Build history of the part. All positions in model axes, mm. Face numbers are marked on the shaded views. A direction names the side the tool comes from. Give positions to 0.01 mm unless a question says otherwise; leave off trailing zeros. Write each loop counter-clockwise with the first axis right and the second up, starting at its lowest first coordinate (ties: lowest second). Pieces come first, ordered by that corner, then holes. Notation, with made-up numbers: (-35.5, -39.5) - (17.5, -39.5) arc R15 ccw to (17.5, -17.5) - close; hole circle Ø6 at (-13, -14.75). An arc over 180 degrees is marked (long way). Use one line per item in the form item = value. Start each with the question number.
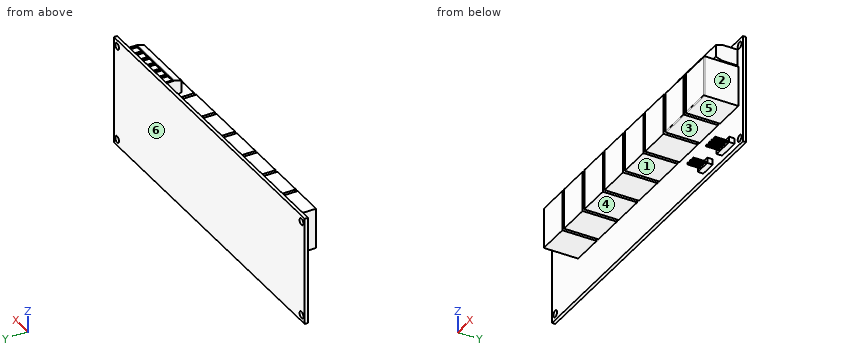
from build123d import *

# Parameters (mm, degrees)
F0_W      = 154.432
F0_H      = 50.419
F0_R      = 1.5113
F1_DEPTH  = 1.524
F2_W      = 14.986
F2_H      = 18.796
F3_DEPTH  = 15.875
F4_R      = 0.381
F5_W      = 30.226
F5_H      = 7.62
F6_DEPTH  = 10.16
F7_SIZE2  = 1.016
F7_SIZE   = 3.175
F8_W      = 4.064
F8_H      = 5.08
F9_DEPTH  = 0.508
F10_W     = 7.62
F10_H     = 2.54
F10_W_2   = 10.16
F11_DEPTH = 2.54
F12_W     = 0.635
F12_H     = 0.635
F13_DEPTH = 5.715


with BuildPart() as f1:
    # F0 (on Front) → F1 (new body)
    with BuildSketch(Plane.XZ):
        Rectangle(F0_W, F0_H)
        with Locations((-74.549, -22.2885)):
            Circle(F0_R, mode=Mode.SUBTRACT)
        with Locations((74.549, -22.2885)):
            Circle(F0_R, mode=Mode.SUBTRACT)
        with Locations((-74.549, 22.2885)):
            Circle(F0_R, mode=Mode.SUBTRACT)
        with Locations((74.549, 22.2885)):
            Circle(F0_R, mode=Mode.SUBTRACT)
    extrude(amount=F1_DEPTH)

    # F2 (on face) → F3 (join)
    with BuildSketch(Plane.XZ.offset(1.524)):
        with Locations((49.7205, 3.1115)):
            Rectangle(F2_W, F2_H)
        with Locations((66.1035, 3.1115)):
            Rectangle(F2_W, F2_H)
        with Locations((33.3375, 3.1115)):
            Rectangle(F2_W, F2_H)
        with Locations((16.9545, 3.1115)):
            Rectangle(F2_W, F2_H)
        with Locations((0.5715, 3.1115)):
            Rectangle(F2_W, F2_H)
        with Locations((-15.8115, 3.1115)):
            Rectangle(F2_W, F2_H)
        with Locations((-32.1945, 3.1115)):
            Rectangle(F2_W, F2_H)
        with Locations((-48.5775, 3.1115)):
            Rectangle(F2_W, F2_H)
    extrude(amount=F3_DEPTH)

    # F4
    f4_edges = [f1.edges().sort_by_distance(p)[0] for p in [
        (42.2275, -17.399, 3.1115),
        (49.7205, -17.399, -6.2865),
        (57.2135, -17.399, 3.1115),
        (49.7205, -17.399, 12.5095),
        (58.6105, -17.399, 3.1115),
        (66.1035, -17.399, -6.2865),
        (73.5965, -17.399, 3.1115),
        (66.1035, -17.399, 12.5095),
    ]]
    fillet(f4_edges, radius=F4_R)

    # F5 (on face) → F6 (join)
    with BuildSketch(Plane.XZ.offset(1.524)):
        with Locations((57.912, 17.2085)):
            Rectangle(F5_W, F5_H)
    extrude(amount=F6_DEPTH)

    # F7
    f7_edges = [f1.edges().sort_by_distance(p)[0] for p in [
        (57.912, -11.684, 21.0185),
        (57.912, -11.684, 13.3985),
    ]]
    chamfer(f7_edges, length=F7_SIZE, length2=F7_SIZE2)

    # F8 (on face) → F9 (cut)
    with BuildSketch(Plane.XY.offset(21.0185)):
        with Locations((45.5295, -5.461)):
            Rectangle(F8_W, F8_H)
        with Locations((50.4825, -5.461)):
            Rectangle(F8_W, F8_H)
        with Locations((55.4355, -5.461)):
            Rectangle(F8_W, F8_H)
        with Locations((60.3885, -5.461)):
            Rectangle(F8_W, F8_H)
        with Locations((65.3415, -5.461)):
            Rectangle(F8_W, F8_H)
        with Locations((70.2945, -5.461)):
            Rectangle(F8_W, F8_H)
    extrude(amount=-F9_DEPTH, mode=Mode.SUBTRACT)

    # F10 (on face) → F11 (join)
    with BuildSketch(Plane.XZ.offset(1.524)):
        with Locations((49.022, -21.3995)):
            Rectangle(F10_W, F10_H)
        with Locations((65.532, -21.3995)):
            Rectangle(F10_W_2, F10_H)
    extrude(amount=F11_DEPTH)

    # F12 (on face) → F13 (join)
    with BuildSketch(Plane.XZ.offset(4.064)):
        with Locations((62.2935, -21.3995)):
            Rectangle(F12_W, F12_H)
        with Locations((64.4525, -21.3995)):
            Rectangle(F12_W, F12_H)
        with Locations((66.6115, -21.3995)):
            Rectangle(F12_W, F12_H)
        with Locations((68.7705, -21.3995)):
            Rectangle(F12_W, F12_H)
        with Locations((51.08575, -21.3995)):
            Rectangle(F12_W, F12_H)
        with Locations((49.022, -21.3995)):
            Rectangle(F12_W, F12_H)
        with Locations((46.95825, -21.3995)):
            Rectangle(F12_W, F12_H)
    extrude(amount=F13_DEPTH)


solid = f1.part
(1) Cut at B-B, the plane x = -43.5. Give the cut face in (y, z).
(2) Two-plate mould, pull along Z, no slides. Class the marked faces 4, 5 and 6: +Z half, -Z half, draft (parallel to the pull), parting line (faces both ways), or undercut.
(3) Wall check: line 1 (Y direction, x = 5, z = 19); line 2 (Z direction, x = -14.5, y = -1.75); line 3 (Y direction, x = 58, z = 16). Give the ranges that are in metal, low to high. Write a range as from..to.
(4) Pin check, flat tips, straight feed: pin 1 Ø4 at (x, z) = (-9, -12.5) entering from -Y; pin 2 Ø1.7 at (x, z) = (57.5, 16) entering from -Y; pin 3 Ø0.7 at (y, z) = (-6.5, -21.5) entering from -X. Stop position of each tip, or through.
(5) Cut at A-A, the plane y = -13. State how many separate pieces and enclosed holes the cut face has, then the cut area to 3 significant figures.
(6) Cut at D-D, the plane x = -62. Give the cut face in (y, z).
(7) Which spindle directions (+Z, -Z, +X, -X, +Y, -Y) get a long thin tool onto all of the face, cutting with end or side? Do the marked faces 1, 2 and 3. Say none if no direction does.
(8) Cut at C-C, the plane z = -8. Give the cut face in (x, y), then the cut area to 3 significant figures.
Solution:
q1.outline = (-17.4, -6.29) - (-1.52, -6.29) - (-1.52, -25.21) - (0, -25.21) - (0, 25.21) - (-1.52, 25.21) - (-1.52, 12.51) - (-17.4, 12.51) - close
q2.face_4 = -Z half
q2.face_5 = undercut
q2.face_6 = draft
q3.line_1 = -1.52..0
q3.line_2 = -6.29..12.51
q3.line_3 = -11.68..0
q4.pin_1 = -1.52
q4.pin_2 = -11.68
q4.pin_3 = 46.64
q5.separate_pieces = 8
q5.enclosed_holes = 0
q5.area = 2,250 mm2
q6.outline = (-1.52, -25.21) - (0, -25.21) - (0, 25.21) - (-1.52, 25.21) - close
q7.face_1 = -Z, +X, -X, -Y
q7.face_2 = +Z, -Z, +X, -Y
q7.face_3 = +X, -X, -Y
q8.outline = (-77.22, -1.52) - (77.22, -1.52) - (77.22, 0) - (-77.22, 0) - close
q8.area = 235 mm2
